Check sheet for the modelled part. Datum: model origin and axes. Units: mm. Face numbers are marked on the shaded views. A direction names the side the tool comes from. Round coordinates to 2 decimals unless told otherwise and drop trailing zeros. Loops run counter-clockwise (first coordinate to the right, second up) from the corner with the lowest first, then second, coordinate; pieces in that order, holes last. Notation, with made-up numbers: (47, -30.75) -> (105, -30.75) arc R23 ccw to (105, 4.25) -> close; hole circle Ø11 at (40, -16.75). An arc over 180 degrees is marked (long way). Use one line per item in the form item = value. Start each with the question number.
(1) Sectioned sample at A-A (y = 10.5). Record the cut outline in (x, z).
(2) Set-up check for the marked faces 1, 2 and 3: record each of +Z, -Z, +X, -X, +Y, -Y from which the full face is reachable in a straight line by a thin tool's end or side.
(3) Sectioned sample at D-D (x = 0). Record the cut outline in (y, z).
(4) Sectioned sample at B-B (x = 9). Record the cut outline in (y, z), and give its area (3 significant figures).
(5) Material ranges on probe 1 along Y at (x, z) = (9, -1); probe 2 along Y at (x, z) = (-7.25, -4.25); probe 3 along Z at (x, y) = (1, 2), recorded low to high. Write a range as [from, to].
(6) Go/stop test with flat-tipped pins: pin 1 (3 mm diameter, centred on x = -7, z = 2.5, fed in from -Y); pin 2 (3.5 mm diameter, centred on x = -3, z = -2.5, fed in from +Y); pin 3 (8 mm diameter, centred on x = 5, y = -8.5, fed in from -Z); pin 4 (4 mm diameter, centred on y = 3.5, z = 0.5, fed in from +X). Record where each tip stops, or that it passes through.
(7) Sectioned sample at C-C (y = -4). Record the cut outline in (x, z), and give its area (3 significant figures).
from build123d import *

# Parameters (mm, degrees)
F1_DEPTH = 2
F3_DEPTH = 26
F4_R     = 4
F5_DEPTH = 15
F6_SIZE  = 1


with BuildPart() as f1:
    # F0 (on Front) → F1 (new body)
    with BuildSketch(Plane.XZ):
        with BuildLine():
            ThreePointArc((9.4344444444, -1.6435504327), (10.3469512901, -1.0371702957), (10.7, 0))
            ThreePointArc((10.7, 0), (10.3469512901, 1.0371702957), (9.4344444444, 1.6435504327))
            Line((9.4344444444, 1.6435504327), (-6.407798527, 5.8311763854))
            ThreePointArc((-6.407798527, 5.8311763854), (-8.5124333236, 5.6159080306), (-9.9516775266, 4.0652938892))
            ThreePointArc((-9.9516775266, 4.0652938892), (-10.5485314952, 2.0714688736), (-10.75, 0))
            ThreePointArc((-10.75, 0), (-10.5485314952, -2.0714688736), (-9.9516775266, -4.0652938892))
            ThreePointArc((-9.9516775266, -4.0652938892), (-8.5124333236, -5.6159080306), (-6.407798527, -5.8311763854))
            Line((-6.407798527, -5.8311763854), (9.4344444444, -1.6435504327))
        make_face()
    extrude(amount=F1_DEPTH)

    # F2 (on face) → F3 (join)
    with BuildSketch(Plane.XZ.offset(2)):
        with BuildLine():
            ThreePointArc((9.4344444444, -1.6435504327), (10.3469512901, -1.0371702957), (10.7, 0))
            ThreePointArc((10.7, 0), (10.3469512901, 1.0371702957), (9.4344444444, 1.6435504327))
            ThreePointArc((9.4344444444, 1.6435504327), (7.3, 0), (9.4344444444, -1.6435504327))
        make_face()
    extrude(amount=F3_DEPTH)

    # F4 (on face) → F5 (join)
    with BuildSketch(Plane(origin=(0, 0, 0), x_dir=(-1, 0, 0), z_dir=(0, 1, 0))):
        Circle(F4_R)
    extrude(amount=F5_DEPTH)

    # F6
    f6_edges = [f1.edges().sort_by_distance(p)[0] for p in [
        (4, 15, 0),
    ]]
    chamfer(f6_edges, length=F6_SIZE)


solid = f1.part
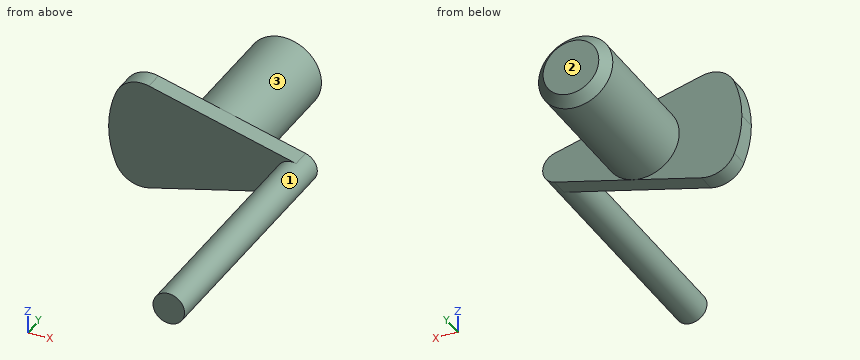
Checks:
q1.outline = circle Ø8 at (0, 0)
q2.face_1 = -Y
q2.face_2 = +Z, -Z, +X, -X, +Y
q2.face_3 = +Y
q3.outline = (-2, -4.14) -> (0, -4.14) -> (0, -4) -> (14, -4) -> (15, -3) -> (15, 3) -> (14, 4) -> (0, 4) -> (0, 4.14) -> (-2, 4.14) -> close
q4.outline = (-28, -1.7) -> (-2, -1.7) -> (-2, -1.76) -> (0, -1.76) -> (0, 1.76) -> (-2, 1.76) -> (-2, 1.7) -> (-28, 1.7) -> close
q4.area = 95.4 mm2
q5.probe_1 = [-28, 0]
q5.probe_2 = [-2, 0]
q5.probe_3 = [-3.87, 3.87]
q6.pin_1 = -2
q6.pin_2 = 15
q6.pin_3 = -1.7
q6.pin_4 = 4
q7.outline = circle Ø3.4 at (9, 0)
q7.area = 9.08 mm2
